```python
from build123d import *

# Parameters (mm, degrees)
SKETCH1_W            = 66
SKETCH1_H            = 56
BASE_DEPTH           = 3
SKETCH4_W            = 66
SKETCH4_H            = 56
SKETCH4_W_2          = 58
SKETCH4_H_2          = 48
WALL1_DEPTH          = 21
WALL2_START          = -21
SKETCH8_W            = 62
SKETCH8_H            = 52
SKETCH8_W_2          = 58
SKETCH8_H_2          = 48
WALL2_DEPTH          = 2
PCBWALL_START        = -3
SKETCH9_W            = 48
SKETCH9_H            = 38
SKETCH9_W_2          = 44
SKETCH9_H_2          = 34
PCBWALL_DEPTH        = 4
SKETCH10_R           = 1.2
MOUNTING_HOLE_DEPTH  = 4
SKETCH11_W           = 66
SKETCH11_H           = 56
EXTENDED_BASE_DEPTH  = 10
HEAD_START           = 28
SKETCH12_W           = 20
SKETCH12_H           = 4
HEAD_BAND_SLOT_DEPTH = 77.104053883
CLIPS_START          = 28
SKETCH13_W           = 8
SKETCH13_H           = 8
CLIPS_DEPTH          = 3
FILLET2_R            = 2.5


with BuildPart() as part:
    # Sketch1 → Base (new body)
    with BuildSketch(Plane(origin=(0, 0, 0), x_dir=(1, 0, 0), z_dir=(0, 1, 0))):
        Rectangle(SKETCH1_W, SKETCH1_H)
    extrude(amount=-BASE_DEPTH)

    # Sketch4 → Wall1 (add)
    with BuildSketch(Plane(origin=(0, 0, 0), x_dir=(1, 0, 0), z_dir=(0, 1, 0))):
        Rectangle(SKETCH4_W, SKETCH4_H)
        Rectangle(SKETCH4_W_2, SKETCH4_H_2, mode=Mode.SUBTRACT)
    extrude(amount=-WALL1_DEPTH)

    # Sketch8 → Wall2 (cut)
    with BuildSketch(Plane(origin=(0, 0, 0), x_dir=(1, 0, 0), z_dir=(0, 1, 0)).offset(WALL2_START)):
        Rectangle(SKETCH8_W, SKETCH8_H)
        Rectangle(SKETCH8_W_2, SKETCH8_H_2, mode=Mode.SUBTRACT)
    extrude(amount=WALL2_DEPTH, mode=Mode.SUBTRACT)

    # Sketch9 → PCBWall (add)
    with BuildSketch(Plane(origin=(0, 0, 0), x_dir=(1, 0, 0), z_dir=(0, 1, 0)).offset(PCBWALL_START)):
        Rectangle(SKETCH9_W, SKETCH9_H)
        Rectangle(SKETCH9_W_2, SKETCH9_H_2, mode=Mode.SUBTRACT)
    extrude(amount=-PCBWALL_DEPTH)

    # Sketch10 → Mounting hole (cut)
    with BuildSketch(Plane(origin=(0, 0, 0), x_dir=(1, 0, 0), z_dir=(0, 1, 0))):
        with Locations(Location((14.7, 13.1, 0), (0, 0, 270))):
            Circle(SKETCH10_R)
    extrude(amount=-MOUNTING_HOLE_DEPTH, mode=Mode.SUBTRACT)

    # Sketch11 → Extended Base (add)
    with BuildSketch(Plane(origin=(0, 0, 0), x_dir=(1, 0, 0), z_dir=(0, 1, 0))):
        Rectangle(SKETCH11_W, SKETCH11_H)
    extrude(amount=EXTENDED_BASE_DEPTH)

    # Sketch12 → Head Band Slot (cut, through all)
    with BuildSketch(Plane.XY.offset(HEAD_START)):
        with Locations((0, 5)):
            Rectangle(SKETCH12_W, SKETCH12_H)
    extrude(amount=-HEAD_BAND_SLOT_DEPTH, mode=Mode.SUBTRACT)

    # Sketch13 → Clips (add)
    with BuildSketch(Plane.XY.offset(CLIPS_START)):
        with Locations((-19, -12)):
            Rectangle(SKETCH13_W, SKETCH13_H)
        with Locations((19, -12)):
            Rectangle(SKETCH13_W, SKETCH13_H)
    clips = extrude(amount=CLIPS_DEPTH)

    # Clips2: Clips across plane
    add(clips.mirror(Plane.XY))

    # Fillet2
    fillet2_edges = [part.edges().sort_by_distance(p)[0] for p in [
        (-23, -12, 31),
        (-19, -16, 31),
        (-15, -12, 31),
        (-19, -8, 31),
        (15, -12, 31),
        (19, -16, 31),
        (23, -12, 31),
        (19, -8, 31),
        (15, -12, -31),
        (19, -8, -31),
        (23, -12, -31),
        (19, -16, -31),
        (-23, -12, -31),
        (-19, -8, -31),
        (-15, -12, -31),
        (-19, -16, -31),
    ]]
    fillet(fillet2_edges, radius=FILLET2_R)


solid = part.part
```
Build history of the part. All positions in model axes, mm. A direction names the side the tool comes from. Coordinates: 2 decimals unless noted, no trailing zeros. Order: outer loops, then holes, each group sorted by start corner. A loop starts at its lowest first (then second) coordinate and runs counter-clockwise, first axis right, second up.
Item 1: Saw through at A-A on x = -9. List the corners of the cut face in (y, z).
Filled in:
outline: (-21, -28) - (3, -28) - (3, 28) - (-21, 28) - (-21, 26) - (-19, 26) - (-19, 24) - (-3, 24) - (-3, 19) - (-7, 19) - (-7, 17) - (-3, 17) - (-3, -17) - (-7, -17) - (-7, -19) - (-3, -19) - (-3, -24) - (-19, -24) - (-19, -26) - (-21, -26) - close; (7, -28) - (10, -28) - (10, 28) - (7, 28) - close
Item 2: Drill centre lines: L1, parallel to Z at x = 18.5, y = -4; L2, parallel to X at y = -4.5, z = -16.5; L3, parallel to X at y = -1.3, z = -13.1. Where is each one in solid material? Low to high.
Filled in:
L1: z = -28 to -24, -19 to -17, 17 to 19, 24 to 28
L2: x = -33 to -29, -24 to -22, 22 to 24, 29 to 33
L3: x = -33 to 13.5, 15.9 to 33
Item 3: Mould opens along Z. For faces 4 (the flat face through (19, -12, 31)), 5 (the flat face through (-33, -6, 0)), 6 (the flat face through (0, -5, 19)), 7 (the flat face through (29, -11, 0)) say: released by +Z, released by -Z, zero draft, split by the parting line, or undercut.
Filled in:
face 4: released by +Z
face 5: zero draft
face 6: undercut
face 7: undercut
Item 4: Saw through at B-B on z = 3. List the corners of the cut face in (x, y).
Filled in:
outline: (-33, -21) - (-31, -21) - (-31, -19) - (-29, -19) - (-29, -3) - (-24, -3) - (-24, -7) - (-22, -7) - (-22, -3) - (22, -3) - (22, -7) - (24, -7) - (24, -3) - (29, -3) - (29, -19) - (31, -19) - (31, -21) - (33, -21) - (33, 10) - (-33, 10) - close; hole (-10, 3) - (10, 3) - (10, 7) - (-10, 7) - close
Item 5: Saw through at D-D on z = -13.1. List the corners of the cut face in (x, y), then the cut area to 3 significant figures.
Filled in:
outline: (-33, -21) - (-31, -21) - (-31, -19) - (-29, -19) - (-29, -3) - (-24, -3) - (-24, -7) - (-22, -7) - (-22, -3) - (13.5, -3) - (13.5, 0) - (15.9, 0) - (15.9, -3) - (22, -3) - (22, -7) - (24, -7) - (24, -3) - (29, -3) - (29, -19) - (31, -19) - (31, -21) - (33, -21) - (33, 10) - (-33, 10) - close; hole (-10, 3) - (10, 3) - (10, 7) - (-10, 7) - close
area: 923 mm2
Item 6: Saw through at C-C on z = -21. List the corners of the cut face in (x, y).
Filled in:
outline: (-33, -21) - (-31, -21) - (-31, -19) - (-29, -19) - (-29, -3) - (29, -3) - (29, -19) - (31, -19) - (31, -21) - (33, -21) - (33, 10) - (-33, 10) - close; hole (-10, 3) - (10, 3) - (10, 7) - (-10, 7) - close
Item 7: Tool access for faces 1 (the cylindrical face through (-15.436, -11.944, -29.911)), 2 (the flat face through (0, -5, 17)), 3 (the cylindrical face through (-18.944, -8.436, 29.911)): list every direction of +Z, -Z, +X, -X, +Y, -Y with a clear straight run to the whole face (end or side of a thin tool).
Filled in:
face 1: -Z, +Y, -Y
face 2: -Y
face 3: +Z, +X, -X, +Y
Item 8: Drop flat-ended pins along their axis: pin 1 Ø4.5 at (x, y) = (1, -5) entering from +Z; pin 2 Ø1.6 at (x, y) = (-10, -20) entering from -Z; pin 3 Ø2.5 at (x, z) = (15, -13) entering from -Y. Give the stop position or say it passes through.
Filled in:
pin 1: stops at z = 28
pin 2: stops at z = -28
pin 3: stops at y = -3
